Verification items for the finished model (mm, model axes). A direction names the side the tool comes from. Coordinates: 2 decimals unless noted, no trailing zeros. Write each loop counter-clockwise with the first axis right and the second up, starting at its lowest first coordinate (ties: lowest second). Pieces come first, ordered by that corner, then holes. Notation, with made-up numbers: M 39,52.25 L 54,52.25 A32 cw 54,86.25 Z; hole C -3,86 d4. An arc over 180 degrees is marked long. One line per item, written item: value.
```python
from build123d import *

# Parameters (mm, degrees)
SKETCH_2_R      = 2
SKETCH_2_W      = 15
SKETCH_2_H      = 5
EXTRUDE_1_DEPTH = 2
SKETCH_1_W      = 15
SKETCH_1_H      = 5
SKETCH_1_R      = 2
EXTRUDE_2_DEPTH = 2


with BuildPart() as part:
    # 草图2 → 凸台-拉伸1 (new body)
    # profile 1 of 2: a face of its own
    with BuildSketch(Plane(origin=(0, 0, 0), x_dir=(1, 0, 0), z_dir=(0, 1, 0))):
        with BuildLine():
            ThreePointArc((-7.5, 5), (0, 12.5), (7.5, 5))
            Line((7.5, 5), (-7.5, 5))
        make_face()
        with Locations(Location((0, 7.5, 0), (0, 0, 270))):
            Circle(SKETCH_2_R, mode=Mode.SUBTRACT)
    # profile 2 of 2: a face of its own
    with BuildSketch(Plane(origin=(0, 0, 0), x_dir=(1, 0, 0), z_dir=(0, 1, 0))):
        with Locations((0, 2.5)):
            Rectangle(SKETCH_2_W, SKETCH_2_H)
    extrude(amount=EXTRUDE_1_DEPTH)

    # 草图1 → 凸台-拉伸2 (add)
    # profile 1 of 2: a face of its own
    with BuildSketch(Plane.XY):
        with Locations((0, 2.5)):
            Rectangle(SKETCH_1_W, SKETCH_1_H)
    # profile 2 of 2: a face of its own
    with BuildSketch(Plane.XY):
        with BuildLine():
            ThreePointArc((-7.5, 5), (0, 12.5), (7.5, 5))
            Line((7.5, 5), (-7.5, 5))
        make_face()
        with Locations((0, 8)):
            Circle(SKETCH_1_R, mode=Mode.SUBTRACT)
    extrude(amount=-EXTRUDE_2_DEPTH)


solid = part.part
```
Item 1: Cross-section at C-C, the plane y = 2.25. Enter the section's corners in (x, z), and give its area (3 significant figures).
The answers:
outline: M -7.5,-2 L 7.5,-2 L 7.5,0 L -7.5,0 Z
area: 30.0 mm²
Item 2: Scan lines: line 1 (Y direction, x = 0, z = -0.5); line 2 (Y direction, x = 0, z = -11.25); line 3 (Z direction, x = -6.5, y = 2.5). Record each from-to range of solid material in increasing order.
The answers:
line 1: y = 0 to 6, 10 to 12.5
line 2: y = 0 to 2
line 3: z = -2 to 0
Item 3: Cross-section at D-D, the plane z = -11. Enter the section's corners in (x, y), and give its area (3 significant figures).
The answers:
outline: M -4.5,0 L 4.5,0 L 4.5,2 L -4.5,2 Z
area: 18.0 mm²
Item 4: Go/stop test with flat-tipped pins: P1, Ø1.5, axis at x = 5, y = 2.5, coming from the -Z side; P2, Ø5, axis at x = 5, y = 8.5, coming from the -Z side; P3, Ø3, axis at y = 2, z = -10, coming from the +X side. Record where each tip stops, or that it passes through.
The answers:
P1: stops at z = -11.04
P2: stops at z = -2
P3: stops at x = 6.63
Item 5: Draft check along Z on faces 3 (the face through (7.5, 1, -2)), 4 (the face through (-1.2, 1, -9.1)), 5 (the face through (0, 5, 0)), 6 (the face through (-0.16, 0.99, -12.5)). Enter one of: released by +Z, released by -Z, zero draft, split by the parting line, or undercut.
The answers:
face 3: zero draft
face 4: undercut
face 5: released by +Z
face 6: released by -Z
Item 6: Cross-section at A-A, the plane x = 0. Enter the section's corners in (y, z).
The answers:
outline: M 0,-12.5 L 2,-12.5 L 2,-9.5 L 0,-9.5 Z; M 0,-5.5 L 2,-5.5 L 2,-2 L 6,-2 L 6,0 L 0,0 Z; M 10,-2 L 12.5,-2 L 12.5,0 L 10,0 Z
Item 7: Access from +Z, -Z, +X, -X, +Y, -Y to the whole of each face (thin tool, end or side, straight path). Record for faces 1 (the face through (0, 5, -2)), 2 (the face through (0, 0, -5)).
The answers:
face 1: -Z, +X, -X, +Y
face 2: +Z, -Z, +X, -X, -Y
Item 8: Cross-section at B-B, the plane z = -7.5. Enter the section's corners in (x, y).
The answers:
outline: M -7.07,0 L -2,0 L -2,2 L -7.07,2 Z; M 2,0 L 7.07,0 L 7.07,2 L 2,2 Z
